For this review, take the finished solid that the model builds, in its own axes (mm). A direction names the side the tool comes from. Give positions to 0.01 mm unless a question says otherwise; leave off trailing zeros. Loops run counter-clockwise (first coordinate to the right, second up) from the corner with the lowest first, then second, coordinate; pieces in that order, holes last. Notation, with made-up numbers: (43.25, 51.25) - (99.25, 51.25) arc R20 cw to (99.25, 70.25) - close; hole circle Ø7 at (0, 19). An arc over 180 degrees is marked (long way). Answer as CSV lines item,"result".
from build123d import *

# Parameters (mm, degrees)
BOSS_EXTRUDE3_DEPTH = 5
SKETCH3_W           = 40
SKETCH3_H           = 49
SKETCH3_W_2         = 34
SKETCH3_H_2         = 43
BOSS_EXTRUDE4_DEPTH = 10.5
SKETCH1_W           = 34
SKETCH1_H           = 43
BOSS_EXTRUDE5_DEPTH = 3
BOSS_EXTRUDE6_DEPTH = 9.5
SKETCH6_R           = 2
CUT_EXTRUDE1_DEPTH  = 3
CIRPATTERN1_COUNT   = 3
SKETCH8_R           = 5
CUT_EXTRUDE2_DEPTH  = 9.5


with BuildPart() as part:
    # Sketch4 → Boss-Extrude3 (new body)
    with BuildSketch(Plane(origin=(0, 0, 0), x_dir=(1, 0, 0), z_dir=(0, 1, 0))):
        with BuildLine():
            Line((6.323055165, 7.747191322), (17.313841595, 47))
            Line((17.313841595, 47), (11, 47))
            Line((11, 47), (11, 54.120862841))
            Line((11, 54.120862841), (-1.380656992, 9.904230726))
            ThreePointArc((-1.380656992, 9.904230726), (-2.696299255, -9.629640197), (6.323055165, 7.747191322))
        make_face()
    boss_extrude3 = extrude(amount=BOSS_EXTRUDE3_DEPTH)

    # Sketch3 → Boss-Extrude4 (add)
    with BuildSketch(Plane(origin=(0, 0, 0), x_dir=(1, 0, 0), z_dir=(0, 1, 0))):
        with Locations((31, 71.5)):
            Rectangle(SKETCH3_W, SKETCH3_H)
        with Locations((31, 71.5)):
            Rectangle(SKETCH3_W_2, SKETCH3_H_2, mode=Mode.SUBTRACT)
    boss_extrude4 = extrude(amount=BOSS_EXTRUDE4_DEPTH)

    # Sketch1 → Boss-Extrude5 (add)
    with BuildSketch(Plane(origin=(0, 0, 0), x_dir=(1, 0, 0), z_dir=(0, 1, 0))):
        with Locations((31, 71.5)):
            Rectangle(SKETCH1_W, SKETCH1_H)
    boss_extrude5 = extrude(amount=BOSS_EXTRUDE5_DEPTH)

    # Sketch7 → Boss-Extrude6 (add)
    with BuildSketch(Plane(origin=(0, 10.5, 0), x_dir=(1, 0, 0), z_dir=(0, 1, 0))):
        Polygon((14, 50), (14, 59), (11, 59), (11, 47), (51, 47), (51, 96), (11, 96), (11, 84), (14, 84), (14, 93), (48, 93), (48, 50), align=None)
    boss_extrude6 = extrude(amount=BOSS_EXTRUDE6_DEPTH)

    # Sketch6 → Cut-Extrude1 (cut)
    with BuildSketch(Plane(origin=(14, 0, 0), x_dir=(0, 0, -1), z_dir=(1, 0, 0))):
        with Locations((55.5, 8.5)):
            Circle(SKETCH6_R)
        with Locations((87.5, 8.5)):
            Circle(SKETCH6_R)
    cut_extrude1 = extrude(amount=-CUT_EXTRUDE1_DEPTH, mode=Mode.SUBTRACT)

    # CirPattern1: Boss-Extrude3, Boss-Extrude4, Boss-Extrude5, Boss-Extrude6, Cut-Extrude1 ×3 about axis
    cirpattern1_axis = Axis((0, 0, 0), (0, 1, 0))
    for i in range(1, CIRPATTERN1_COUNT):
        add(boss_extrude3.rotate(cirpattern1_axis, i * 360 / CIRPATTERN1_COUNT))
        add(boss_extrude4.rotate(cirpattern1_axis, i * 360 / CIRPATTERN1_COUNT))
        add(boss_extrude5.rotate(cirpattern1_axis, i * 360 / CIRPATTERN1_COUNT))
        add(boss_extrude6.rotate(cirpattern1_axis, i * 360 / CIRPATTERN1_COUNT))
        add(cut_extrude1.rotate(cirpattern1_axis, i * 360 / CIRPATTERN1_COUNT), mode=Mode.SUBTRACT)

    # Sketch8 → Cut-Extrude2 (cut)
    with BuildSketch(Plane(origin=(0, 5, 0), x_dir=(1, 0, 0), z_dir=(0, 1, 0))):
        Circle(SKETCH8_R)
    extrude(amount=-CUT_EXTRUDE2_DEPTH, mode=Mode.SUBTRACT)


solid = part.part
1) Insertion check: P1, Ø8, axis at x = 38, y = 4.5, coming from the +Z side; P2, Ø5, axis at y = 5.5, z = -40, coming from the -X side; P3, Ø2.5, axis at y = 8.5, z = -87.5, coming from the -X side. Each pin has a flat end and moves straight along its axis. Give the tip position at first contact, or say it passes through.
From the geometry:
P1,"stops at z = 83.14"
P2,"stops at x = 6.36"
P3,"stops at x = 48"
2) Machinability: for faces 5 (the flat face through (-67.718, 7.638, 26.395)), 6 (the flat face through (17.6, 2.46, 23.72)), 7 (the flat face through (38.18, 11.38, 77.47)), 8 (the flat face through (11, 8, -72)), 9 (the flat face through (51, 10, -71)), which of the approach directions +Z, -Z, +X, -X, +Y, -Y give a long, thin tool a straight path to every point of the face, cutting with its end or side? Answer none if there is none.
From the geometry:
face 5,"+Z, +Y"
face 6,"+Y, -Y"
face 7,"+Y"
face 8,"-Z, -X, +Y"
face 9,"-Z, +X, +Y, -Y"
3) Draft analysis for pull direction X (two halves, no side actions). For faces 1 (the flat face through (-98.78, 9.86, 20.91)), 2 (the flat face through (-68.7, 9.5, 23.5)), 3 (the flat face through (56.72, 7.64, 45.45)), 4 (the flat face through (31, 10, -96)), state which applies: pulls with the +X half, pulls with the -X half, needs draft (parallel to the pull), parting line crosses it, or undercut.
From the geometry:
face 1,"pulls with the -X half"
face 2,"undercut"
face 3,"pulls with the +X half"
face 4,"needs draft"
4) Consider section C-C on z = -70. Write out the cut boundary in (x, y).
From the geometry:
outline,"(11, 0) - (51, 0) - (51, 20) - (48, 20) - (48, 3) - (14, 3) - (14, 10.5) - (11, 10.5) - close"
5) Consider section B-B on y = 14.75. Count the separate pieces of the cut face and the enclosed holes in it, and give its area (3 significant figures).
From the geometry:
separate pieces,"3"
enclosed holes,"0"
area,"1,270 mm^2"
6) Wall thickness on line 1 (X direction, y = 7.75, z = -67); line 2 (Y direction, x = 12.1, z = -87.5); line 3 (X direction, y = 4.25, z = 24.5): over which ranges is each line inside the solid? List them lowest first. Write a range as from..to.
From the geometry:
line 1,"x = 11..14, 48..51"
line 2,"y = 0..6.5, 10.5..20"
line 3,"x = -96.71..-93.24, -70.44..-64.44, 18.36..29.55"
7) Consider section A-A on x = 29. Write out the cut boundary in (y, z).
From the geometry:
outline,"(0, -96) - (20, -96) - (20, -93) - (3, -93) - (3, -50) - (20, -50) - (20, -47) - (0, -47) - close; (0, 23.94) - (5, 23.94) - (5, 35.38) - (0, 35.38) - close; (0, 43.77) - (20, 43.77) - (20, 49.77) - (3, 49.77) - (3, 72.17) - (20, 72.17) - (20, 75.63) - (0, 75.63) - close"
8) Consider section D-D on x = 62.5. Write out the cut boundary in (y, z).
From the geometry:
outline,"(0, 48.79) - (10.5, 48.79) - (10.5, 52.25) - (3, 52.25) - (3, 77.75) - (20, 77.75) - (20, 83.75) - (0, 83.75) - close"
